from build123d import *

# Parameters (mm, degrees)
F0_R     = 9.5758
F1_DEPTH = 31.75
F2_R     = 7.9629
F3_DEPTH = 25.4
F4_R     = 4.7625
F5_DEPTH = 25.4
F6_R     = 3.1496
F7_DEPTH = 25.4


with BuildPart() as f1:
    # F0 (on Front) → F1 (new body)
    with BuildSketch(Plane.XZ):
        Circle(F0_R)
    extrude(amount=-F1_DEPTH)

    # F2 (on face) → F3 (cut)
    with BuildSketch(Plane(origin=(0, 31.75, 0), x_dir=(-1, 0, 0), z_dir=(0, 1, 0))):
        Circle(F2_R)
    extrude(amount=-F3_DEPTH, mode=Mode.SUBTRACT)

    # F4 (on face) → F5 (join)
    with BuildSketch(Plane.XZ):
        Circle(F4_R)
    extrude(amount=F5_DEPTH)

    # F6 (on face) → F7 (cut)
    with BuildSketch(Plane.XZ.offset(25.4)):
        Circle(F6_R)
    extrude(amount=-F7_DEPTH, mode=Mode.SUBTRACT)


solid = f1.part
CAD build for the part. Positions are in the model's coordinates, mm. A direction names the side the tool comes from. Give positions to 0.01 mm unless a question says otherwise; leave off trailing zeros. Write each loop counter-clockwise with the first axis right and the second up, starting at its lowest first coordinate (ties: lowest second). Pieces come first, ordered by that corner, then holes. Notation, with made-up numbers: M -35,52 L 20,52 A35 cw 20,87 Z; hole C -32.5,45.5 d6. An arc over 180 degrees is marked long. Put each result on its own line as item: value. Start each with the question number.
(1) Band-saw the part on B-B, the plane z = 0. Write the cut outline in (x, y), and give its area (3 significant figures).
(2) Which spindle directions (+Z, -Z, +X, -X, +Y, -Y) get a long thin tool onto all of the face, cutting with end or side? Do faces 1 (the face through (0, 6.35, 0)), 2 (the face through (-2.499, -12.878, -1.916)), 3 (the face through (-1.13, -25.4, -3.11)). Say none if no direction does.
(3) Band-saw the part on C-C, the plane y = -11.5. Write the cut outline in (x, z) (1 decimal).
(4) Mould opens along Z. For faces 4 (the face through (0, 0, 0)), 5 (the face through (9.134, 15.653, 2.876)), 6 (the face through (-2.3, 0, 4.4)) say: +Z half, -Z half, draft (parallel to the pull), parting line (faces both ways), or undercut.
(5) Band-saw the part on A-A, the plane x = 0. Write the cut outline in (y, z), and give its area (3 significant figures).
(6) Flat gauge pins, fed straight in: pin 1 Ø5 at (x, y) = (5.5, -0.5) entering from +Z; pin 2 Ø8 at (x, z) = (-3.5, -1) entering from +Y; pin 3 Ø10 at (x, y) = (2.5, -6.5) entering from +Z. Where does each tip first touch, or does it go through?
(7) Band-saw the part on D-D, the plane z = 7.25. Write the cut outline in (x, y), and give its area (3 significant figures).
(8) Probe L1, parallel to Z at x = 0, y = 22.5; L2, parallel to Z at x = 0, y = -9; L3, parallel to Y at x = 3.75, z = -0.5. List the from-to ranges inside material, lowest first.
Response values:
1. outline: M -9.58,0 L -4.76,0 L -4.76,-25.4 L -3.15,-25.4 L -3.15,0 L 3.15,0 L 3.15,-25.4 L 4.76,-25.4 L 4.76,0 L 9.58,0 L 9.58,31.75 L 7.96,31.75 L 7.96,6.35 L -7.96,6.35 L -7.96,31.75 L -9.58,31.75 Z
1. area: 285 mm2
2. face 1: +Y
2. face 2: -Y
2. face 3: +Z, -Z, +X, -X, -Y
3. outline: C 0,0 d9.5; hole C 0,0 d6.3
4. face 4: undercut
4. face 5: parting line
4. face 6: draft
5. outline: M -25.4,-4.76 L 0,-4.76 L 0,-9.58 L 31.75,-9.58 L 31.75,-7.96 L 6.35,-7.96 L 6.35,7.96 L 31.75,7.96 L 31.75,9.58 L 0,9.58 L 0,4.76 L -25.4,4.76 L -25.4,3.15 L 0,3.15 L 0,-3.15 L -25.4,-3.15 Z
5. area: 285 mm2
6. pin 1: stops at z = 9.08
6. pin 2: stops at y = 6.35
6. pin 3: stops at z = 4.76
7. outline: M -6.26,0 L 6.26,0 L 6.26,31.75 L 3.29,31.75 L 3.29,6.35 L -3.29,6.35 L -3.29,31.75 L -6.26,31.75 Z
7. area: 230 mm2
8. L1: z = -9.58 to -7.96, 7.96 to 9.58
8. L2: z = -4.76 to -3.15, 3.15 to 4.76
8. L3: y = -25.4 to 6.35
